Autodesk Inventor part; units mm, degrees
ref_plane "YZ Plane" through (0, 0, 0) normal (1, 0, 0) x (0, 1, 0)
ref_plane "XZ Plane" through (0, 0, 0) normal (0, 1, 0) x (-1, 0, 0)
ref_plane "XY Plane" through (0, 0, 0) normal (0, 0, 1) x (1, 0, 0)
sketch "Sketch1" plane through (0, 0, 0) normal (0, 0, 1) x (1, 0, 0)
  circle A0 centre (-3.2439, -112.6362) radius 2.7 construction
  circle A1 centre (-3.2439, -130.6362) radius 2.7 construction
  line L0 (49.7615, -342.4426) -> (49.7615, 314.6303) construction
  line L1 (-11.2439, -109.7245) -> (-11.2439, -135.255)
  line L2 (-11.2439, -109.7245) -> (19.7615, -72.7737)
  line L3 (19.7615, -72.7737) -> (49.7615, -72.7737)
  circle A2 centre (-3.2439, -112.6362) radius 3
  circle A3 centre (-3.2439, -130.6362) radius 3
  line L4 (-11.2439, -135.255) -> (34.7615, -161.8162)
  line L5 (34.7615, -161.8162) -> (49.7615, -161.8162)
  line L6 (110.7669, -109.7245) -> (110.7669, -135.255)
  line L7 (110.7669, -109.7245) -> (79.7615, -72.7737)
  line L8 (79.7615, -72.7737) -> (49.7615, -72.7737)
  circle A4 centre (102.7669, -112.6362) radius 3
  circle A5 centre (102.7669, -130.6362) radius 3
  line L9 (110.7669, -135.255) -> (64.7615, -161.8162)
  line L10 (64.7615, -161.8162) -> (49.7615, -161.8162)
  point P0 (0, 0)
  dimension "d0" = 6
  dimension "d1" = 6
  dimension "d8" = 8
  dimension "d16" = 30
  dimension "d17" = 15
  dimension "d18" = 60
  dimension "d19" = 40
  dimension "d20" = 8
  dimension "d21" = 8
extrude "Plate1" add sketch "Sketch1" along normal blind 3
fillet "Fillet1" radius 4 6 edges at (-11.2439, -135.255, 1.5) (-11.2439, -109.7245, 1.5) (110.7669, -109.7245, 1.5) (110.7669, -135.255, 1.5) (64.7615, -161.8162, 1.5) (34.7615, -161.8162, 1.5)
sketch "Sketch2" plane through (0, 0, 3) normal (0, 0, 1) x (1, 0, 0)
  arc A0 (19.774, -118.0434) -> (18.9211, -121.2485) centre (16.9316, -119.0031) ccw
  arc A1 (80.0915, -120.6614) -> (80.0915, -117.3448) centre (82.5915, -119.0031) ccw
  arc A2 (47.082, -94.8758) -> (52.441, -94.8758) centre (49.7615, -96.225) ccw
  line L0 (3.7561, -107.7275) -> (3.7561, -132.1292)
  line L1 (3.7561, -107.7275) -> (17.5274, -91.3156)
  line L2 (17.5274, -91.3156) -> (30.8475, -118.3156)
  line L3 (30.8475, -118.3156) -> (30.8475, -131.9856)
  line L4 (30.8475, -131.9856) -> (24.0125, -143.8242)
  line L5 (24.0125, -143.8242) -> (3.7561, -132.1292)
  line L6 (24.6949, -82.7737) -> (38.0151, -109.7737)
  line L7 (38.0151, -109.7737) -> (61.508, -109.7737)
  line L8 (19.7615, -72.7737) -> (79.7615, -72.7737)
  line L9 (61.508, -109.7737) -> (74.8281, -82.7737)
  line L10 (74.8281, -82.7737) -> (24.6949, -82.7737)
  line L11 (-10.308, -108.6092) -> (19.7615, -72.7737)
  line L12 (33.8333, -161.2803) -> (-9.2439, -136.4097)
  line L13 (-11.2439, -132.9456) -> (-11.2439, -111.1803)
  arc A3 (63.6897, -161.8162) -> (65.6897, -161.2803) centre (63.6897, -157.8162) ccw
  line L14 (19.7615, -72.7737) -> (63.6897, -161.8162) construction
  line L15 (17.5274, -91.3156) -> (24.6949, -82.7737) construction
  line L16 (38.0151, -109.7737) -> (30.8475, -118.3156) construction
  line L17 (49.7615, -82.7737) -> (49.7615, -72.7737) construction
  line L18 (79.7615, -72.7737) -> (109.8311, -108.6092)
  line L19 (35.8333, -161.8162) -> (63.6897, -161.8162)
  line L20 (79.7615, -72.7737) -> (35.8333, -161.8162) construction
  line L21 (95.7669, -107.7275) -> (95.7669, -132.1292)
  line L22 (95.7669, -107.7275) -> (81.9957, -91.3156)
  line L23 (81.9957, -91.3156) -> (68.6755, -118.3156)
  line L24 (68.6755, -118.3156) -> (68.6755, -131.9856)
  line L25 (68.6755, -131.9856) -> (75.5105, -143.8242)
  line L26 (75.5105, -143.8242) -> (95.7669, -132.1292)
  line L27 (42.3946, -131.9856) -> (32.6728, -148.8242)
  line L28 (32.6728, -148.8242) -> (65.3755, -148.8242)
  line L29 (65.3755, -148.8242) -> (55.6538, -131.9856)
  line L30 (55.6538, -131.9856) -> (42.3946, -131.9856)
  line L31 (30.8475, -131.9856) -> (68.6755, -131.9856) construction
  line L32 (24.0125, -143.8242) -> (32.6728, -148.8242) construction
  line L33 (65.3755, -148.8242) -> (75.5105, -143.8242) construction
  point P0 (0, 0)
  point P1 (37.5337, -140.4049)
  dimension "d22" = 10
  dimension "d23" = 15
  dimension "d24" = 27
  dimension "d25" = 10.2071
  dimension "d26" = 10.2071
  dimension "d27" = 10.2071
  dimension "d28" = 10
extrude "Cut1" cut sketch "Sketch2" against normal blind 3
fillet "Fillet2" radius 2 22 edges at (19.7615, -72.7737, 1.5) (79.7615, -72.7737, 1.5) (17.5274, -91.3156, 1.5) (3.7561, -107.7275, 1.5) (3.7561, -132.1292, 1.5) (24.0125, -143.8242, 1.5) (30.8475, -131.9856, 1.5) (30.8475, -118.3156, 1.5) (74.8281, -82.7737, 1.5) (24.6949, -82.7737, 1.5) (38.0151, -109.7737, 1.5) (61.508, -109.7737, 1.5) (81.9957, -91.3156, 1.5) (68.6755, -118.3156, 1.5) (68.6755, -131.9856, 1.5) (75.5105, -143.8242, 1.5) (95.7669, -132.1292, 1.5) (95.7669, -107.7275, 1.5) (55.6538, -131.9856, 1.5) (42.3946, -131.9856, 1.5) (32.6728, -148.8242, 1.5) (65.3755, -148.8242, 1.5)
equation "\"d26\" = d25"
equation "\"d27\" = d25"
equation "\"d10\" = Thickness"
equation "\"BendRadius\" = Thickness"
equation "\"BendReliefWidth\" = Thickness"
equation "\"BendReliefDepth\" = 0.5 * Thickness"
equation "\"CornerReliefSize\" = 4 * Thickness"
equation "\"MinimumRemnant\" = 2 * Thickness"
equation "\"TransitionRadius\" = BendRadius"
equation "\"JacobiRadiusSize\" = BendRadius"
equation "\"GapSize\" = Thickness"
properties part number "JawMount"
CAD build for the part. Positions are in the model's coordinates, mm. A direction names the side the tool comes from. Round coordinates to 2 decimals unless told otherwise and drop trailing zeros. Order: outer loops, then holes, each group sorted by start corner. A loop starts at its lowest first (then second) coordinate and runs counter-clockwise, first axis right, second up.
Item 1: Probe line 1 along X through (y, z) = (-119.5, 1.35); line 2 along X through (y, z) = (-106.5, 0.25); line 3 along Y through (x, z) = (50, 2.25). List the from-to ranges inside material, lowest first.
Item 2: Tool access for faces 5 (the face through (24.68, -105.81, 1.52)), 6 (the face through (11.99, -148.67, 1.48)): list every direction of +Z, -Z, +X, -X, +Y, -Y with a clear straight run to the whole face (end or side of a thin tool).
Item 3: Saw through at A-A on y = -103. Write the cut outline in (x, z), then the cut area to 3 significant figures.
Item 4: Mould opens along X. For faces 1 (the face through (-11, -109.8, 1.5)), 2 (the face through (49, -148.824, 2)), 3 (the face through (-3.63, -115.61, 1.48)), 4 (the face through (110.2, -135, 1.5)) say: pulls with the +X half, pulls with the -X half, needs draft (parallel to the pull), parting line crosses it, or undercut.
Item 5: Saw through at C-C on z = 1.5. State how many separate pieces and enclosed holes the cut face has, then the cut area to 3 significant figures.
Item 6: Saw through at B-B on x = 92. Write the cut outline in (y, z), then the cut area to 3 significant figures.
Item 7: Pin check, flat tips, straight feed: pin 1 (1.5 mm diameter, centred on y = -98.5, z = 1.5, fed in from +X); pin 2 (1 mm diameter, centred on y = -139.5, z = 1, fed in from +X). Stop position of each tip, or through.
Reported:
1. line 1: x = -11.24 to 3.76, 30.85 to 68.68, 95.77 to 110.77
1. line 2: x = -8.54 to 4.79, 25.02 to 36.4, 63.12 to 74.5, 94.74 to 108.06
1. line 3: y = -161.82 to -148.82, -131.99 to -109.77, -82.77 to -72.77
2. face 5: +Z, -Z
2. face 6: +Z, -Z, -X, -Y
3. outline: (-5.6, 0) - (7.72, 0) - (7.72, 3) - (-5.6, 3) - close; (23.29, 0) - (34.67, 0) - (34.67, 3) - (23.29, 3) - close; (64.85, 0) - (76.23, 0) - (76.23, 3) - (64.85, 3) - close; (91.8, 0) - (105.12, 0) - (105.12, 3) - (91.8, 3) - close
3. area: 148 mm2
4. face 1: pulls with the -X half
4. face 2: undercut
4. face 3: undercut
4. face 4: pulls with the +X half
5. separate pieces: 1
5. enclosed holes: 8
5. area: 5,080 mm2
6. outline: (-146.09, 0) - (-134.3, 0) - (-134.3, 3) - (-146.09, 3) - close; (-103.24, 0) - (-87.36, 0) - (-87.36, 3) - (-103.24, 3) - close
6. area: 83.0 mm2
7. pin 1: stops at x = 101.98
7. pin 2: stops at x = 104.28
